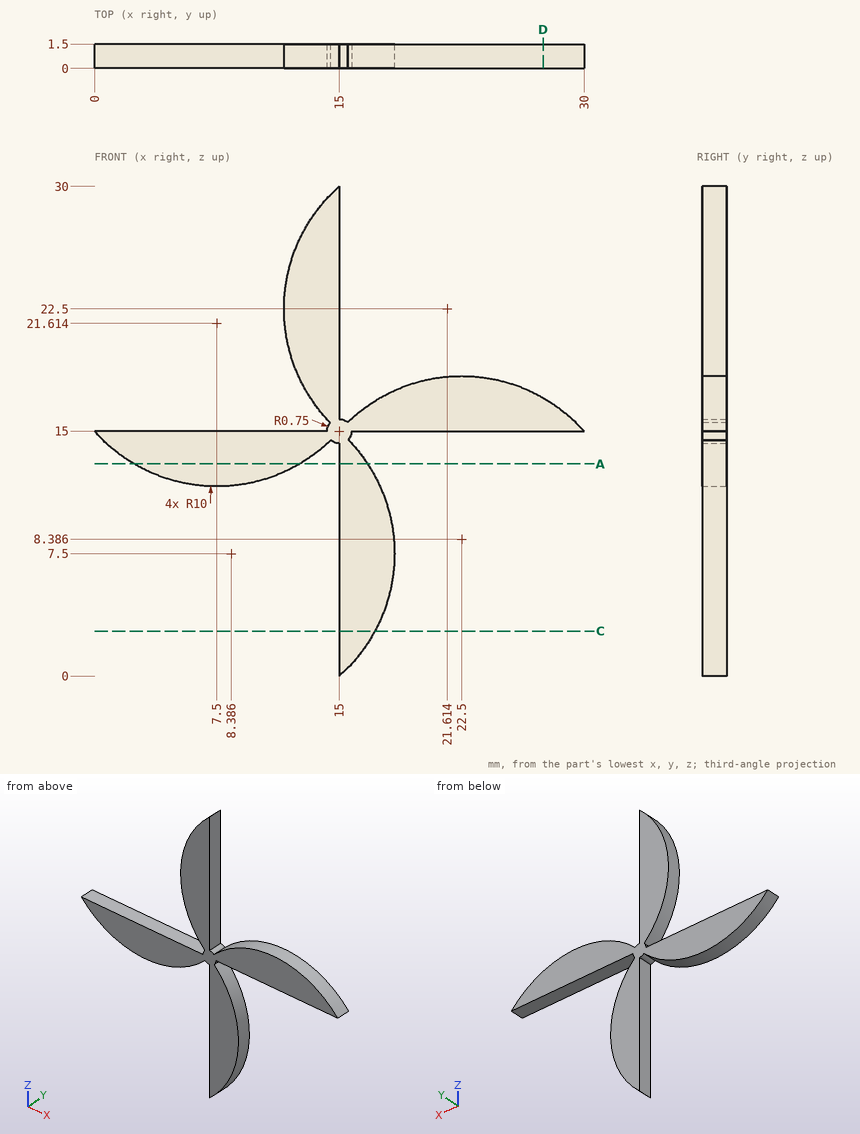
Geometry: see drawing. Coordinates: mm, zero at the bounding-box minimum. Coordinates: 2 decimals unless noted, no trailing zeros. Loops run counter-clockwise (first coordinate to the right, second up) from the corner with the lowest first, then second, coordinate; pieces in that order, holes last. Notation, with made-up numbers: M -26,75.5 L -4,75.5 A13 cw -4,79.5 Z; hole C 25.25,32 d9. An arc over 180 degrees is marked long. Put each result on its own line as item: value. Start each with the question number.
1) Cut plane C-C on z = 2.75. Return the cut outline in (x, y) (1 decimal).
2) Ray query, L1, parallel to X at y = 0.25, z = 13.25 (1 decimal); L2, parallel to X at y = 0.3, z = 16.75 (1 decimal); L3, parallel to Z at x = 13, y = 1.1 (1 decimal). Return the intervals inside material, ascending. Write a range as from..to.
3) Cut plane D-D on x = 27.5. Return the cut outline in (y, z).
4) Cut plane A-A on z = 13. Return the cut outline in (x, y).
5) Contact query for a flat-ended pin moving along its axis: pin 1 Ø0.8 at (x, y) = (6.5, 1) entering from +Z. Output: stop coordinate, or through.
The answers:
1. outline: M 15,0 L 17.2,0 L 17.2,1.5 L 15,1.5 Z
2. L1: x = 2..13, 15..16.6
2. L2: x = 13.4..15, 17..28
2. L3: z = 13.3..15, 17.4..27.6
3. outline: M 0,15 L 1.5,15 L 1.5,17.05 L 0,17.05 Z
4. outline: M 2.42,0 L 12.58,0 L 12.58,1.5 L 2.42,1.5 Z; M 15,0 L 16.74,0 L 16.74,1.5 L 15,1.5 Z
5. pin 1: stops at z = 15
